```python
from build123d import *

# Parameters (mm, degrees)
BOSS_EXTRU_1_DEPTH      = 9
D_GAGEMENT_M31_D        = 3.4
ENL_V_MAT_EXTRU_1_DEPTH = 2.5
D_GAGEMENT_M32_D        = 3.4
ENL_V_MAT_EXTRU_2_DEPTH = 2.5
CONG_1_R                = 2


with BuildPart() as part:
    # Esquisse1 → Boss.-Extru.1 (new body)
    with BuildSketch(Plane(origin=(0, 0, 0), x_dir=(1, 0, 0), z_dir=(0, 1, 0))):
        with BuildLine():
            Line((-99, 2.5), (-77, 2.5))
            ThreePointArc((-77, 2.5), (-72, 7.5), (-67, 2.5))
            Line((-67, 2.5), (-5, 2.5))
            ThreePointArc((-5, 2.5), (0, 7.5), (5, 2.5))
            Line((5, 2.5), (67, 2.5))
            ThreePointArc((67, 2.5), (72, 7.5), (77, 2.5))
            Line((77, 2.5), (99, 2.5))
            Line((99, 2.5), (99, -2.5))
            Line((99, -2.5), (-99, -2.5))
            Line((-99, -2.5), (-99, 2.5))
        make_face()
    extrude(amount=BOSS_EXTRU_1_DEPTH)

    # Dégagement M31 (through all)
    with Locations(Plane(origin=(0, 9, 0), x_dir=(1, 0, 0), z_dir=(0, 1, 0))):
        with Locations((-72, 2.5), (0, 2.5), (72, 2.5)):
            Hole(D_GAGEMENT_M31_D / 2)

    # Esquisse5 → Enlèv. mat.-Extru.1 (cut)
    with BuildSketch(Plane.XZ):
        Polygon((70.41228676, -5.25), (73.58771324, -5.25), (75.175426481, -2.5), (73.58771324, 0.25), (70.41228676, 0.25), (68.824573519, -2.5), align=None)
        Polygon((-1.58771324, -5.25), (1.58771324, -5.25), (3.175426481, -2.5), (1.58771324, 0.25), (-1.58771324, 0.25), (-3.175426481, -2.5), align=None)
        Polygon((-73.58771324, -5.25), (-70.41228676, -5.25), (-68.824573519, -2.5), (-70.41228676, 0.25), (-73.58771324, 0.25), (-75.175426481, -2.5), align=None)
    extrude(amount=-ENL_V_MAT_EXTRU_1_DEPTH, mode=Mode.SUBTRACT)

    # Dégagement M32 (through all)
    with Locations(Plane.XY.offset(2.5)):
        with Locations((-91, 4.5), (-30.333333333, 4.5), (30.333333333, 4.5), (91, 4.5)):
            Hole(D_GAGEMENT_M32_D / 2)

    # Esquisse9 → Enlèv. mat.-Extru.2 (cut)
    with BuildSketch(Plane(origin=(0, 0, -2.5), x_dir=(-1, 0, 0), z_dir=(0, 0, -1))):
        Polygon((-89.41228676, 7.25), (-92.58771324, 7.25), (-94.175426481, 4.5), (-92.58771324, 1.75), (-89.41228676, 1.75), (-87.824573519, 4.5), align=None)
        Polygon((-28.745620093, 7.25), (-31.921046574, 7.25), (-33.508759814, 4.5), (-31.921046574, 1.75), (-28.745620093, 1.75), (-27.157906853, 4.5), align=None)
        Polygon((31.921046574, 7.25), (28.745620093, 7.25), (27.157906853, 4.5), (28.745620093, 1.75), (31.921046574, 1.75), (33.508759814, 4.5), align=None)
        Polygon((92.58771324, 7.25), (89.41228676, 7.25), (87.824573519, 4.5), (89.41228676, 1.75), (92.58771324, 1.75), (94.175426481, 4.5), align=None)
    extrude(amount=-ENL_V_MAT_EXTRU_2_DEPTH, mode=Mode.SUBTRACT)

    # Congé1
    cong_1_edges = [part.edges().sort_by_distance(p)[0] for p in [
        (-77, 4.5, -2.5),
        (-67, 4.5, -2.5),
        (-5, 4.5, -2.5),
        (5, 4.5, -2.5),
        (67, 4.5, -2.5),
        (77, 4.5, -2.5),
    ]]
    fillet(cong_1_edges, radius=CONG_1_R)


solid = part.part
```
Check sheet for the modelled part. Datum: model origin and axes. Units: mm. A direction names the side the tool comes from. Round coordinates to 2 decimals unless told otherwise and drop trailing zeros. Order: outer loops, then holes, each group sorted by start corner. A loop starts at its lowest first (then second) coordinate and runs counter-clockwise, first axis right, second up. Notation, with made-up numbers: (-16, 87) -> (43, 87) arc R22 cw to (43, 104) -> close; hole circle Ø3 at (9, 59). An arc over 180 degrees is marked (long way). One line per item, written item: value. Start each with the question number.
Q1. Set-up check for faces 1 (the face through (1.4, 2.5, -1.2)), 2 (the face through (-36, 4, -2.5)), 3 (the face through (89.6, 5.8, 0)): record each of +Z, -Z, +X, -X, +Y, -Y from which the full face is reachable in a straight line by a thin tool's end or side.
Q2. Thickness scan on line 1 (X direction, y = 4.25, z = 2); line 2 (X direction, y = 6.25, z = -4); line 3 (X direction, y = 5.5, z = -6.5). Record the ranges inside material, lowest first.
Q3. Mould release check, pull along Z, two halves, no side actions. Record for faces 4 (the face through (29, 6, 0)), 5 (the face through (-70.6, 2.5, -1.2)), 6 (the face through (1, 0, 1)), 7 (the face through (-70.3, 5.7, -2.57)): pulls with the +Z half, pulls with the -Z half, needs draft (parallel to the pull), parting line crosses it, or undercut.
Q4. Cross-section at C-C (x = -46). Record the boundary of the cut face in (y, z).
Q5. Cross-section at B-B (x = 91). Record the boundary of the cut face in (y, z), and give its area (4 significant figures).
Q6. Gauge pin test, flat ends, axial feed: pin 1 Ø1 at (y, z) = (1, -5.5) entering from -X; pin 2 Ø2.5 at (x, y) = (90, 3.5) entering from -Z; pin 3 Ø2 at (y, z) = (3, -4) entering from +X. Record the tip position at first contact, or that the pin passes through.
Q7. Cross-section at A-A (x = 0). Record the boundary of the cut face in (y, z), and give its area (4 significant figures).
Completed:
1. face 1: -Y
1. face 2: -Z, +Y, -Y
1. face 3: -Z
2. line 1: x = -99 to -92.68, -89.32 to -32.01, -28.65 to 28.65, 32.01 to 89.32, 92.68 to 99
2. line 2: x = -76.77 to -72.8, -71.2 to -67.23, -4.77 to -0.8, 0.8 to 4.77, 67.23 to 71.2, 72.8 to 76.77
2. line 3: x = -75 to -69, -3 to 3, 69 to 75
3. face 4: pulls with the -Z half
3. face 5: undercut
3. face 6: needs draft
3. face 7: undercut
4. outline: (0, -2.5) -> (9, -2.5) -> (9, 2.5) -> (0, 2.5) -> close
5. outline: (0, -2.5) -> (1.75, -2.5) -> (1.75, 0) -> (2.8, 0) -> (2.8, 2.5) -> (0, 2.5) -> close; (6.2, 0) -> (7.25, 0) -> (7.25, -2.5) -> (9, -2.5) -> (9, 2.5) -> (6.2, 2.5) -> close
5. area: 22.75 mm²
6. pin 1: stops at x = -76.33
6. pin 2: stops at z = 0
6. pin 3: stops at x = 77.39
7. outline: (0, -7.5) -> (9, -7.5) -> (9, -4.2) -> (2.5, -4.2) -> (2.5, -5.25) -> (0, -5.25) -> close; (0, 0.25) -> (2.5, 0.25) -> (2.5, -0.8) -> (9, -0.8) -> (9, 2.5) -> (0, 2.5) -> close
7. area: 54.15 mm²
